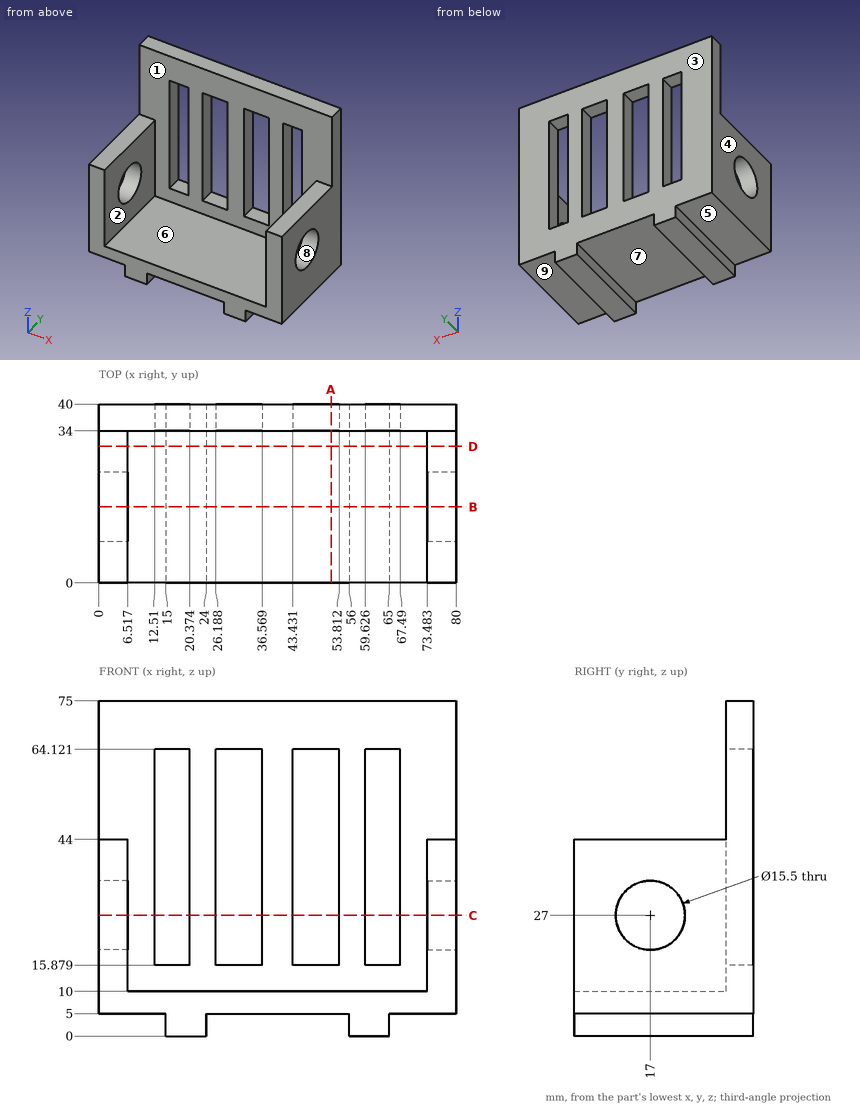
Study the drawing (mm; zero at the part's minimum x, y, z) and answer. A direction names the side the tool comes from. Coordinates: 2 decimals unless noted, no trailing zeros. Write each loop counter-clockwise with the first axis right and the second up, starting at its lowest first coordinate (ties: lowest second). Pieces come first, ordered by that corner, then holes. Notation, with made-up numbers: M 68,72 L 82,72 A33 cw 82,106 Z; hole C -31,4 d4. An arc over 180 degrees is marked long. Use one line per item in the form item = value.
Item 1: Find section D-D, the plane y = 30.5. Give the vertices of the cut face in (x, z), plus the area to 3 significant figures.
Model answer:
outline = M 0,5 L 15,5 L 15,0 L 24,0 L 24,5 L 56,5 L 56,0 L 65,0 L 65,5 L 80,5 L 80,44 L 73.48,44 L 73.48,10 L 6.52,10 L 6.52,44 L 0,44 Z
area = 933 mm2
Item 2: Find section C-C, the plane z = 27. Give the number of separate pieces and of enclosed holes in the cut face, plus the area to 3 significant figures.
Model answer:
separate_pieces = 7
enclosed_holes = 0
area = 502 mm2
Item 3: Find the intervals of material crossed by probe 1 along X at (y, z) = (35, 29); probe 2 along X at (y, z) = (32, 40); probe 3 along Z at (x, y) = (76, 17), in increasing order.
Model answer:
probe_1 = 0 to 12.51, 20.37 to 26.19, 36.57 to 43.43, 53.81 to 59.63, 67.49 to 80
probe_2 = 0 to 6.52, 73.48 to 80
probe_3 = 5 to 19.25, 34.75 to 44
Item 4: Find section A-A, the plane x = 52. Give the vertices of the cut face in (y, z).
Model answer:
outline = M 0,5 L 40,5 L 40,15.88 L 34,15.88 L 34,10 L 0,10 Z; M 34,64.12 L 40,64.12 L 40,75 L 34,75 Z
Item 5: The mould has two halves that part along X. Classify the marked faces 1, 2, 3 and 4: released by +X, released by -X, zero draft, split by the parting line, or undercut.
Model answer:
face_1 = undercut
face_2 = undercut
face_3 = zero draft
face_4 = released by -X
Item 6: Given P1, Ø5, axis at x = 56, z = 37, coming from the -Y side; P2, Ø4, axis at x = 25.5, y = 20, coming from the +Z side; P3, Ø1.8, axis at x = 47.5, y = 37.5, coming from the -Z side, each flat-ended and moving along its own axis, determine where each tip first touches the part or whether it passes through.
Model answer:
P1 = 34
P2 = 10
P3 = 5
Item 7: For the marked faces 5, 6, 7, 8 and 9, determine the directions among +Z, -Z, +X, -X, +Y, -Y from which every point of the face is accessible in a straight line to the end or side of a thin tool.
Model answer:
face_5 = -Z, -X, +Y, -Y
face_6 = +Z, -Y
face_7 = -Z, +Y, -Y
face_8 = +X, -X
face_9 = -Z, +X, +Y, -Y
Item 8: Find section B-B, the plane y = 17. Give the vertices of the cut face in (x, z), plus the area to 3 significant figures.
Model answer:
outline = M 0,5 L 15,5 L 15,0 L 24,0 L 24,5 L 56,5 L 56,0 L 65,0 L 65,5 L 80,5 L 80,19.25 L 73.48,19.25 L 73.48,10 L 6.52,10 L 6.52,19.25 L 0,19.25 Z; M 0,34.75 L 6.52,34.75 L 6.52,44 L 0,44 Z; M 73.48,34.75 L 80,34.75 L 80,44 L 73.48,44 Z
area = 731 mm2
